The model under review builds one solid part; all positions refer to its coordinate system, in mm. A direction names the side the tool comes from. Round coordinates to 2 decimals unless told otherwise and drop trailing zeros. Order: outer loops, then holes, each group sorted by start corner. A loop starts at its lowest first (then second) coordinate and runs counter-clockwise, first axis right, second up. Notation, with made-up numbers: M 46,8.25 L 103,8.25 A25 cw 103,22.25 Z; hole C 59.5,-31.75 d9. An arc over 180 degrees is marked long. Answer as a JSON object with one key per item and string values. Group by question number.
1) Consider section B-B, the plane y = 5.5. Write out the cut boundary in (x, z).
2) Consider section D-D, the plane z = 1.75. Count the separate pieces of the cut face and the enclosed holes in it, then the cut area to 3 significant figures.
3) The part is to be moulded in two halves that separate along X. For faces 1 (the cylindrical face through (-19.463, 25.373, 3.219)), 2 (the flat face through (25, -28.575, 3)), 3 (the cylindrical face through (-14.15, 39.75, 3.13)), say which applies: +X half, -X half, draft (parallel to the pull), parting line (faces both ways), or undercut.
4) Consider section C-C, the plane x = -38.1. Write out the cut boundary in (y, z) (3 decimals), then the cut area to 3 significant figures.
5) For faces 4 (the flat face through (-63.5, -3, 3)), 5 (the cylindrical face through (-55.44, 24.9, 3.22)), list the 3-axis set-ups (+Z, -Z, +X, -X, +Y, -Y) from which the entire face can be reached by the end or side of a thin tool; tool diameter is ignored.
6) Consider section A-A, the plane x = -69.85. Write out the cut boundary in (y, z) (3 decimals).
7) Insertion check: pin 1 Ø6 at (x, y) = (10.16, 13.38) entering from +Z; pin 2 Ø1.9 at (x, z) = (21.5, 2.5) entering from -Y (3 decimals); pin 3 Ø1.3 at (y, z) = (34.5, 2.5) entering from +X. Each pin has a flat end and moves straight along its axis. Give the tip position at first contact, or say it passes through.
8) To check wall thickness, follow line 1 (Y direction, x = -57.15, z = 1.75) (3 decimals); line 2 (Y direction, x = 57.15, z = 2.75) (3 decimals); line 3 (X direction, y = -21, z = 6). State the ranges of each line that lie inside material, in increasing order.
```python
from build123d import *

# Parameters (mm, degrees)
SKETCH1_W           = 127
SKETCH1_H           = 57.15
SKETCH1_R           = 14.3002
SKETCH1_R_2         = 2.38125
BOSS_EXTRUDE1_DEPTH = 6.35
SKETCH2_R           = 2.38125
CUT_EXTRUDE1_DEPTH  = 70.922121857
FILLET1_R           = 5.08
SKETCH3_R           = 3.175
CUT_EXTRUDE2_DEPTH  = 70.922121857
SKETCH4_R           = 16.51
CUT_EXTRUDE3_DEPTH  = 7.62
SKETCH5_W           = 76.2
SKETCH5_H           = 12.7
BOSS_EXTRUDE2_DEPTH = 6.35
FILLET2_R           = 5.08
SKETCH6_W           = 25.4
SKETCH6_H           = 5.08
BOSS_EXTRUDE3_DEPTH = 6.35
FILLET3_R           = 5.08
SKETCH7_R           = 2.38125
CUT_EXTRUDE4_DEPTH  = 6.35


with BuildPart() as part:
    # Sketch1 → Boss-Extrude1 (new body)
    with BuildSketch(Plane.XY):
        Rectangle(SKETCH1_W, SKETCH1_H)
        with Locations((31.75, 0)):
            Circle(SKETCH1_R, mode=Mode.SUBTRACT)
        with Locations((37.555148495, -24.727722316)):
            Circle(SKETCH1_R_2, mode=Mode.SUBTRACT)
        with Locations((10.16, 13.380280266)):
            Circle(SKETCH1_R_2, mode=Mode.SUBTRACT)
        with Locations((25.944851505, 24.727722316)):
            Circle(SKETCH1_R_2, mode=Mode.SUBTRACT)
        with Locations((53.34, -13.380280266)):
            Circle(SKETCH1_R_2, mode=Mode.SUBTRACT)
    extrude(amount=BOSS_EXTRUDE1_DEPTH)

    # Sketch2 → Cut-Extrude1 (cut, through all)
    with BuildSketch(Plane.XY.offset(6.35)):
        with Locations((57.15, 22.225)):
            Circle(SKETCH2_R)
        with Locations((57.15, -22.225)):
            Circle(SKETCH2_R)
        with Locations((0, 22.225)):
            Circle(SKETCH2_R)
        with Locations((0, -22.225)):
            Circle(SKETCH2_R)
    extrude(amount=-CUT_EXTRUDE1_DEPTH, mode=Mode.SUBTRACT)

    # Fillet1
    fillet1_edges = [part.edges().sort_by_distance(p)[0] for p in [
        (63.5, -28.575, 3.175),
        (63.5, 28.575, 3.175),
    ]]
    fillet(fillet1_edges, radius=FILLET1_R)

    # Sketch3 → Cut-Extrude2 (cut, through all)
    with BuildSketch(Plane.XY.offset(6.35)):
        with Locations((-57.15, 22.225)):
            Circle(SKETCH3_R)
        with Locations((-19.05, 22.225)):
            Circle(SKETCH3_R)
        with Locations(Location((-19.05, -22.225, 0), (0, 0, 180))):
            Circle(SKETCH3_R)
        with Locations(Location((-57.15, -22.225, 0), (0, 0, 180))):
            Circle(SKETCH3_R)
    extrude(amount=-CUT_EXTRUDE2_DEPTH, mode=Mode.SUBTRACT)

    # Sketch4 → Cut-Extrude3 (cut)
    with BuildSketch(Plane.XY.offset(6.35)):
        with Locations((-38.1, 9.525)):
            Circle(SKETCH4_R)
    extrude(amount=-CUT_EXTRUDE3_DEPTH, mode=Mode.SUBTRACT)

    # Sketch5 → Boss-Extrude2 (add)
    with BuildSketch(Plane.XY.offset(6.35)):
        with Locations((-50.8, -34.925)):
            Rectangle(SKETCH5_W, SKETCH5_H)
        with Locations((-50.8, 34.925)):
            Rectangle(SKETCH5_W, SKETCH5_H)
    extrude(amount=-BOSS_EXTRUDE2_DEPTH)

    # Fillet2
    fillet2_edges = [part.edges().sort_by_distance(p)[0] for p in [
        (-12.7, 41.275, 3.175),
        (-12.7, 28.575, 3.175),
        (-12.7, -28.575, 3.175),
        (-12.7, -41.275, 3.175),
    ]]
    fillet(fillet2_edges, radius=FILLET2_R)

    # Sketch6 → Boss-Extrude3 (add)
    with BuildSketch(Plane.XY.offset(6.35)):
        with Locations((-76.2, 26.035)):
            Rectangle(SKETCH6_W, SKETCH6_H)
    extrude(amount=-BOSS_EXTRUDE3_DEPTH)

    # Fillet3
    fillet3_edges = [part.edges().sort_by_distance(p)[0] for p in [
        (-88.9, 41.275, 3.175),
        (-88.9, -41.275, 3.175),
    ]]
    fillet(fillet3_edges, radius=FILLET3_R)

    # Sketch7 → Cut-Extrude4 (cut)
    with BuildSketch(Plane.XY.offset(6.35)):
        with Locations((-82.55, 34.925)):
            Circle(SKETCH7_R)
        with Locations((-82.55, -34.925)):
            Circle(SKETCH7_R)
        with Locations((-69.85, 34.925)):
            Circle(SKETCH7_R)
        with Locations((-69.85, -34.925)):
            Circle(SKETCH7_R)
    extrude(amount=-CUT_EXTRUDE4_DEPTH, mode=Mode.SUBTRACT)


solid = part.part
```
Results list:
{
 "1": {"outline": "M -63.5,0 L -54.11,0 L -54.11,6.35 L -63.5,6.35 Z; M -22.09,0 L 18.55,0 L 18.55,6.35 L -22.09,6.35 Z; M 44.95,0 L 63.5,0 L 63.5,6.35 L 44.95,6.35 Z"},
 "2": {"separate pieces": "1", "enclosed holes": "18", "area": "7,460 mm^2"},
 "3": {"face 1": "undercut", "face 2": "draft", "face 3": "+X half"},
 "4": {"outline": "M -41.275,0 L -6.985,0 L -6.985,6.35 L -41.275,6.35 Z; M 26.035,0 L 41.275,0 L 41.275,6.35 L 26.035,6.35 Z", "area": "315 mm^2"},
 "5": {"face 4": "+Z, -Z, -X", "face 5": "+Z, -Z"},
 "6": {"outline": "M -41.275,0 L -37.306,0 L -37.306,6.35 L -41.275,6.35 Z; M -32.544,0 L -28.575,0 L -28.575,6.35 L -32.544,6.35 Z; M 23.495,0 L 32.544,0 L 32.544,6.35 L 23.495,6.35 Z; M 37.306,0 L 41.275,0 L 41.275,6.35 L 37.306,6.35 Z"},
 "7": {"pin 1": "z = 6.35", "pin 2": "y = -28.575", "pin 3": "x = -12.7"},
 "8": {"line 1": "-41.275 to -25.4, -19.05 to 19.05, 25.4 to 41.275", "line 2": "-28.575 to -24.606, -19.844 to 19.844, 24.606 to 28.575", "line 3": "-63.5 to -60.08, -54.22 to -21.98, -16.12 to -2.04, 2.04 to 55.11, 59.19 to 63.5"}
}
